from build123d import *

# Parameters (mm, degrees)
SKETCH1_W           = 50.8
SKETCH1_H           = 38.1
BOSS_EXTRUDE1_DEPTH = 2.921
SKETCH2_W           = 6.35
SKETCH2_H           = 2.921
CUT_EXTRUDE1_DEPTH  = 63.628546983
SKETCH3_W           = 7.355919967
SKETCH3_H           = 12.7
CUT_EXTRUDE2_DEPTH  = 63.628546983
CUT_EXTRUDE3_DEPTH  = 63.628546983
SKETCH5_W           = 1.5875
SKETCH5_H           = 6.35
CUT_EXTRUDE4_DEPTH  = 63.628546983


with BuildPart() as part:
    # Sketch1 → Boss-Extrude1 (new body)
    with BuildSketch(Plane.XY):
        with Locations((25.4, 17.4625)):
            Rectangle(SKETCH1_W, SKETCH1_H)
    extrude(amount=-BOSS_EXTRUDE1_DEPTH)

    # Sketch2 → Cut-Extrude1 (cut, through all)
    with BuildSketch(Plane.XY):
        with Locations((15.875, 1.4605)):
            Rectangle(SKETCH2_W, SKETCH2_H)
        with Locations((34.925, 1.4605)):
            Rectangle(SKETCH2_W, SKETCH2_H)
    extrude(amount=-CUT_EXTRUDE1_DEPTH, mode=Mode.SUBTRACT)

    # Sketch3 → Cut-Extrude2 (cut, through all)
    with BuildSketch(Plane.XY):
        with Locations((-0.756959983, 17.4625)):
            Rectangle(SKETCH3_W, SKETCH3_H)
    extrude(amount=-CUT_EXTRUDE2_DEPTH, mode=Mode.SUBTRACT)

    # Sketch4 → Cut-Extrude3 (cut, through all)
    with BuildSketch(Plane.XY):
        Polygon((3.175, 19.36115), (6.175375, 19.36115), (6.175375, 21.55825), (9.2075, 21.55825), (9.2075, 19.36115), (10.795, 19.36115), (10.795, 15.56385), (9.2075, 15.56385), (9.2075, 13.36675), (6.175375, 13.36675), (6.175375, 15.56385), (3.175, 15.56385), align=None)
    extrude(amount=-CUT_EXTRUDE3_DEPTH, mode=Mode.SUBTRACT)

    # Sketch5 → Cut-Extrude4 (cut, through all)
    with BuildSketch(Plane.XY):
        with Locations((48.41875, 26.9875)):
            Rectangle(SKETCH5_W, SKETCH5_H)
        with Locations((48.41875, 7.9375)):
            Rectangle(SKETCH5_W, SKETCH5_H)
    extrude(amount=-CUT_EXTRUDE4_DEPTH, mode=Mode.SUBTRACT)


solid = part.part
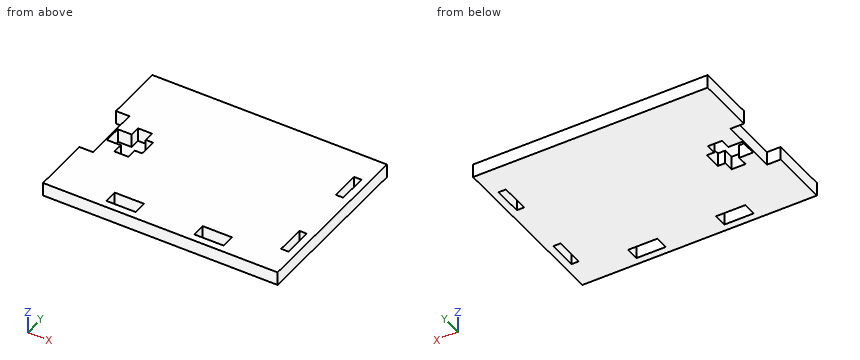
Input: part model. Units: mm. Frame: model coordinates. Round coordinates to 2 decimals unless told otherwise and drop trailing zeros. Loops run counter-clockwise (first coordinate to the right, second up) from the corner with the lowest first, then second, coordinate; pieces in that order, holes last. Notation, with made-up numbers: M -23.5,56 L 28.5,56 A19 cw 28.5,85 Z; hole C 71,76 d8. An arc over 180 degrees is marked long. Answer as CSV lines item,"result". Start each with the question number.
(1) Section C-C, the plane z = -2.15. State how many separate pieces and enclosed holes the cut face has, plus the area to 3 significant figures.
(2) Section B-B, the plane y = 17. Output: boundary loops of the cut face in (x, z) (3 decimals), plus the area to 3 significant figures.
(3) Section A-A, the plane y = 25. Output: boundary loops of the cut face in (x, z) (1 decimal), plus the area to 3 significant figures.
(4) Line query: line 1 (Y direction, x = 49, z = -1.75); line 2 (X direction, y = 1, z = -0.6); line 3 (X direction, y = 11, z = -1.8) (1 decimal). Output: solid intervals per line, ascending. Write a range as [from, to].
(5) First-contact query: pin 1 (0.9 mm diameter, centred on y = 16, z = -1.5, fed in from -X). Flat tip, straight axial feed; report the tip coordinate or a pass-through.
Values found:
1,separate pieces,"1"
1,enclosed holes,"5"
1,area,"1,800 mm²"
2,outline,"M 2.921,-2.921 L 3.175,-2.921 L 3.175,0 L 2.921,0 Z; M 10.795,-2.921 L 50.8,-2.921 L 50.8,0 L 10.795,0 Z"
2,area,"118 mm²"
3,outline,"M 0,-2.9 L 47.6,-2.9 L 47.6,0 L 0,0 Z; M 49.2,-2.9 L 50.8,-2.9 L 50.8,0 L 49.2,0 Z"
3,area,"144 mm²"
4,line 1,"y = [-1.59, 4.76], [11.11, 23.81], [30.16, 36.51]"
4,line 2,"x = [0, 12.7], [19.05, 31.75], [38.1, 50.8]"
4,line 3,"x = [0, 47.6], [49.2, 50.8]"
5,pin 1,"stops at x = 2.92"
